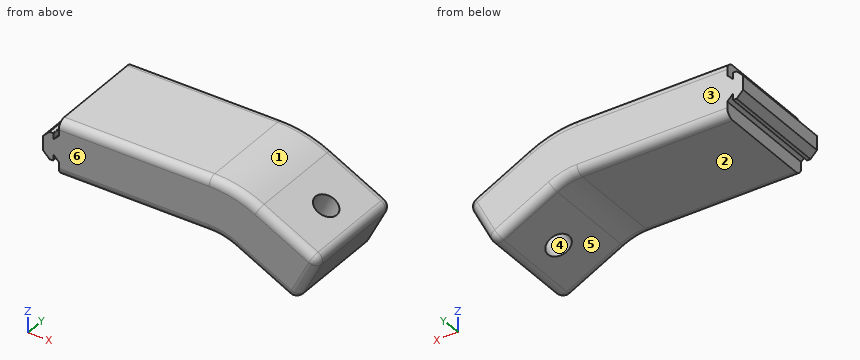
Autodesk Fusion 360 part; units mm, degrees
sketch "Sketch1" plane through (0, 0, 0) normal (0, 1, 0) x (1, 0, 0)
  line L0 (0, 0) -> (55.1984, 0)
  line L1 (64.2782, 2.1799) -> (86.7302, 13.6197)
  line L2 (0, -20) -> (55.1984, -20)
  line L3 (73.358, -15.6403) -> (95.81, -4.2004)
  line L4 (86.7302, 13.6197) -> (95.81, -4.2004)
  line L5 (-2, -12.9989) -> (-2, -14.799)
  line L6 (-2.1998, -14.999) -> (-3.4, -15)
  line L7 (-2, -7) -> (-2, -5.2)
  line L8 (-2.2, -5) -> (-3.4, -5)
  line L9 (-3.4, -5) -> (7.0965, -5) construction
  line L10 (-3.4, -15) -> (7.6345, -15) construction
  line L11 (-5.8, -10) -> (-5.8, -7.4)
  line L12 (-5.8, -10) -> (-5.8, -12.6)
  line L13 (-3.4, -5) -> (-5.8, -7.4)
  line L14 (-3.4, -15) -> (-5.8, -12.6)
  line L15 (0, 0) -> (0, -5)
  line L16 (0, -15) -> (0, -20)
  arc A0 (55.1984, -20) -> (73.358, -15.6403) centre (55.1984, 20) ccw
  arc A1 (55.1984, 0) -> (64.2782, 2.1799) centre (55.1984, 20) ccw
  line L17 (-2, -12.9989) -> (-2, -12.7489)
  line L18 (0, -15) -> (0, -14.75)
  line L19 (-2, -12.7489) -> (0, -14.75)
  line L20 (0, -5) -> (0, -5.25)
  line L21 (-2, -7) -> (-2, -7.25)
  line L22 (-2, -7.25) -> (0, -5.25)
  arc A2 (-2, -5.2) -> (-2.2, -5) centre (-2.2, -5.2) ccw
  arc A3 (-2.1998, -14.999) -> (-2, -14.799) centre (-2.2, -14.799) ccw
  point P0 (60, 0)
  point P1 (-2, -14.9989)
  point P2 (-2, -5)
  dimension "d1" = 153
  dimension "d2" = 30
  dimension "d4" = 1.4
  dimension "d5" = 1.4
  dimension "d7" = 135
  dimension "d8" = 135
  dimension "d10" = 40
  dimension "d11" = 20
  dimension "d18" = 2
  dimension "d19" = 5
  dimension "d20" = 0.25
  dimension "d21" = 0.25
  dimension "d22" = 0.25
  dimension "d23" = 0.25
  dimension "d24" = 0.2
  dimension "d25" = 0.2
extrude "Extrude1" add sketch "Sketch1" along normal blind 40
sketch "Sketch2" plane through (21.4463, 0, 42.0906) normal (0.454, 0, 0.891) x (0.891, 0, -0.454)
  line L0 (58.262, 0) -> (83.4604, 0)
  line L1 (83.4604, 0) -> (83.4604, 40)
  line L2 (83.4604, 40) -> (58.262, 40)
  line L3 (58.262, 40) -> (58.262, 0)
sketch "Sketch3" plane through (12.3664, 0, 24.2705) normal (-0.454, 0, -0.891) x (-0.891, 0, 0.454)
  line L0 (-83.4604, 0) -> (-58.262, 0)
  line L1 (-58.262, 0) -> (-58.262, 40)
  line L2 (-58.262, 40) -> (-83.4604, 40)
  line L3 (-83.4604, 40) -> (-83.4604, 0)
  circle A0 centre (-70.8612, 20) radius 4.35
  dimension "d14" = 8.7
extrude "Extrude2" cut sketch "Sketch3" against normal blind 20 contours A0
fillet "Fillet1" radius 3 16 edges at (27.5992, 40, 20) (64.5362, 40, 18.8948) (84.584, 40, 9.9203) (27.5992, 0, 20) (64.5362, 0, 18.8948) (84.584, 0, 9.9203) (75.5042, 40, -7.8998) (59.8673, 40, -0.5526) (27.5992, 40, 0) (91.2701, 40, -4.7096) (95.81, 20, 4.2004) (86.7302, 20, -13.6197) (91.2701, 0, -4.7096) (27.5992, 0, 0) (59.8673, 0, -0.5526) (75.5042, 0, -7.8998)
Input: part model. Units: mm. Frame: model coordinates. Face numbers are marked on the shaded views. A direction names the side the tool comes from. Coordinates: 2 decimals unless noted, no trailing zeros. Loops run counter-clockwise (first coordinate to the right, second up) from the corner with the lowest first, then second, coordinate; pieces in that order, holes last. Notation, with made-up numbers: M 72.25,35 L 125.25,35 A17 ccw 125.25,61 Z; hole C 30.25,-5.75 d10. An arc over 180 degrees is marked long. Use a Markdown table: item, result. Add a question column.
1) Section C-C, the plane y = 19. Return the cut outline in (x, z).
2) Set-up query: the marked faces 1 and 2. Return all of +Z, -Z, +X, -X, +Y, -Y with unobstructed straight access to the full face (end or side cutting, diameter ignored); none if empty.
3) Pin query (flat end, axial travel): P1, Ø8, axis at y = 19, z = -2, coming from the +X side; P2, Ø8, axis at x = 26.5, y = 21.5, coming from the -Z side; P3, Ø1.3, axis at x = -3, y = 19.5, coming from the -Z side; P4, Ø2, axis at x = 75.5, z = 4.5, coming from the -Y side. Return the tip coordinate at first contact, or that it passes through.
4) Section B-B, the plane x = 11.5. Return the cut outline in (y, z).
5) Section A-A, the plane y = 33. Return the cut outline in (x, z).
6) Line query: L1, parallel to X at y = 17, z = 4; L2, parallel to Y at x = 79.5, z = -8; L3, parallel to X at y = 21, z = -5.5. Output: solid intervals per line, ascending. Write a range as from..to.
7) Draft query along Y for the marked faces 3, 4, 5 and 6. Return one class per face: +Y half, -Y half, draft (parallel to the pull), parting line (faces both ways), or undercut.
Answer below:
| question | item | result |
|---|---|---|
| 1 | outline | M -5.8,7.4 L -3.4,5 L -2.2,5 A0.2 ccw -2,5.2 L -2,7.25 L 0,5.25 L 0,0 L 55.2,0 A20 cw 64.28,-2.18 L 71.73,-5.98 L 80.81,11.84 L 73.36,15.64 A40 ccw 55.2,20 L 0,20 L 0,14.75 L -2,12.75 L -2,14.8 A0.2 ccw -2.2,15 L -3.4,15 L -5.8,12.6 Z; M 79.28,-9.82 L 84.06,-12.26 A3 ccw 88.09,-10.95 L 94.45,1.53 A3 ccw 93.14,5.56 L 88.36,8 Z |
| 2 | face 1 | +Z, +X, +Y, -Y |
| 2 | face 2 | -Z, -X, +Y, -Y |
| 3 | P1 | x = 94.64 |
| 3 | P2 | z = 0 |
| 3 | P3 | z = 5 |
| 3 | P4 | y = 0 |
| 4 | outline | M 0,3 A3 ccw 3,0 L 37,0 A3 ccw 40,3 L 40,17 A3 ccw 37,20 L 3,20 A3 ccw 0,17 Z |
| 5 | outline | M -5.8,7.4 L -3.4,5 L -2.2,5 A0.2 ccw -2,5.2 L -2,7.25 L 0,5.25 L 0,0 L 55.2,0 A20 cw 64.28,-2.18 L 84.06,-12.26 A3 ccw 88.09,-10.95 L 94.45,1.53 A3 ccw 93.14,5.56 L 73.36,15.64 A40 ccw 55.2,20 L 0,20 L 0,14.75 L -2,12.75 L -2,14.8 A0.2 ccw -2.2,15 L -3.4,15 L -5.8,12.6 Z |
| 6 | L1 | 0..78.03, 85.1..94.56 |
| 6 | L2 | 0.28..17.57, 22.43..39.72 |
| 6 | L3 | 70.79..71.98, 81.48..90.87 |
| 7 | face 3 | +Y half |
| 7 | face 4 | undercut |
| 7 | face 5 | draft |
| 7 | face 6 | -Y half |
